from build123d import *

# Parameters (mm, degrees)
F0_W        = 28.575
F0_H        = 25.4
F1_DEPTH    = 3.175
F2_DEPTH    = 6.35
F3_T4_DEPTH = 58.0603739472
F6_DEPTH    = 25.4
F7_DEPTH    = 50.8


# Not quite as in the source:
# - a fillet or chamfer that OpenCascade refuses, or shapes differently, is made with other operations: its cross-section is extruded or revolved along the edge and cut away or added
# - a feature names something its author has since deleted; it is built from what else it names


with BuildPart() as f1:
    # F0 (on Top) → F1 (new body)
    with BuildSketch(Plane.XY):
        with Locations((14.2875, 0)):
            Rectangle(F0_W, F0_H)
        with BuildLine():
            Line((-9.525, -12.7), (0, -12.7))
            Line((0, -12.7), (0, 12.7))
            Line((0, 12.7), (-9.525, 12.7))
            Line((-9.525, 12.7), (-28.575, -4.1005208253))
            ThreePointArc((-28.575, -4.1005208253), (-25.0870430294, -7.374431916), (-21.0470880315, -9.9362869613))
            Line((-21.0470880315, -9.9362869613), (-10.525, -0.6566775598))
            Line((-10.525, -0.6566775598), (-11.1864378278, 0.0933224402))
            Line((-11.1864378278, 0.0933224402), (-21.3967655869, -8.9113402448))
            ThreePointArc((-21.3967655869, -8.9113402448), (-24.4613665471, -6.7728299311), (-27.1481868608, -4.1755232473))
            Line((-27.1481868608, -4.1755232473), (-9.525, 11.3666666667))
            Line((-9.525, 11.3666666667), (-9.525, -12.7))
        make_face()
    extrude(amount=F1_DEPTH)

    # F0 (on Top) → F2 (join)
    with BuildSketch(Plane.XY):
        with BuildLine():
            Line((-9.525, -12.7), (0, -12.7))
            Line((0, -12.7), (0, 12.7))
            Line((0, 12.7), (-9.525, 12.7))
            Line((-9.525, 12.7), (-28.575, -4.1005208253))
            ThreePointArc((-28.575, -4.1005208253), (-25.0870430294, -7.374431916), (-21.0470880315, -9.9362869613))
            Line((-21.0470880315, -9.9362869613), (-10.525, -0.6566775598))
            Line((-10.525, -0.6566775598), (-11.1864378278, 0.0933224402))
            Line((-11.1864378278, 0.0933224402), (-21.3967655869, -8.9113402448))
            ThreePointArc((-21.3967655869, -8.9113402448), (-24.4613665471, -6.7728299311), (-27.1481868608, -4.1755232473))
            Line((-27.1481868608, -4.1755232473), (-9.525, 11.3666666667))
            Line((-9.525, 11.3666666667), (-9.525, -12.7))
        make_face()
    extrude(amount=F2_DEPTH)

    # F3: chamfer of 6.35 on 1 edges, made by hand


with BuildPart() as f3_tool2:
    # F3_s3 → F3_t4 (new body)
    with BuildSketch(Plane.XZ.offset(29.0301869736)):
        Polygon((0, 0), (-6.35, 6.35), (0, 6.35), align=None)
    extrude(amount=-F3_T4_DEPTH)

    split(bisect_by=Plane.XY.offset(3.175), keep=Keep.TOP)


with BuildPart() as f1_1:
    add(f1.part)

    # F3_t1: cut F3_tool2
    add(f3_tool2.part, mode=Mode.SUBTRACT)

    # F5 (on face) → F6 (join)
    with BuildSketch(Plane(origin=(0, 12.7, 0), x_dir=(-1, 0, 0), z_dir=(0, 1, 0))):
        Polygon((3.175, 3.175), (-28.575, 3.175), (-28.575, 0), (9.525, 0), (9.525, 6.35), (6.35, 6.35), align=None)
        Polygon((-28.575, 0), (-28.575, 3.175), (-31.75, 3.175), align=None)
    extrude(amount=-F6_DEPTH)

    # F4 (on face) → F7 (cut)
    with BuildSketch(Plane(origin=(-9.525, 0, 0), x_dir=(0, -1, 0), z_dir=(-1, 0, 0))):
        Polygon((9.9561735988, 0), (12.7, 0), (12.7, 3.175), align=None)
    extrude(amount=-F7_DEPTH, mode=Mode.SUBTRACT)


solid = f1_1.part
Geometry: final body of the model. Coordinates: model frame, mm. A direction names the side the tool comes from. Give positions to 0.01 mm unless a question says otherwise; leave off trailing zeros. Write each loop counter-clockwise with the first axis right and the second up, starting at its lowest first coordinate (ties: lowest second). Pieces come first, ordered by that corner, then holes.
(1) Cut plane B-B, the plane z = 5.75. Return loops of the section in (x, y) (3 decimals), then the cut area to 3 significant figures.
(2) Ray query, line 1 (X direction, y = -4, z = 6) (3 decimals); line 2 (X direction, y = -1.25, z = 0.75) (3 decimals); line 3 (Z direction, x = 5.5, y = -8.5) (3 decimals). Return the intervals inside material, ascending.
(3) Cut plane C-C, the plane x = -4.5. Return loops of the section in (y, z) (3 decimals).
(4) Cut plane D-D, the plane y = 2. Return loops of the section in (x, z) (3 decimals).
(5) Cut plane A-A, the plane y = -7.5. Return loops of the section in (x, z) (3 decimals), then the cut area to 3 significant figures.
(6) Mould query, pull axis Y, two halves, no side actions, for faces 1 (the cylindrical face through (-25.14, -7.333, 3.131)), 2 (the flat face through (6, 2, 0)), 3 (the flat face through (-16.22, -4.346, 3.131)), 4 (the cylindrical face through (-24.421, -6.806, 3.131)). Classes: released by +Y, released by -Y, zero draft, split by the parting line, or undercut.
(7) Access query for faces 5 (the flat face through (-18.46, 3.487, 3.131)), 6 (the flat face through (14, 0, 3.175)), 7 (the flat face through (-9.525, 0, 3)). Directions: +Z, -Z, +X, -X, +Y, -Y. A direction counts if a zero-diameter tool reaches every point of the face in a straight line with its end or side. Return the directions, or none.
(8) First-contact query: P1, Ø10, axis at x = 20.5, y = 5.5, coming from the +Z side (3 decimals). Flat tip, straight axial feed; report the tip coordinate or a pass-through.
Values follow:
1. outline: (-28.575, -4.101) arc R25.4 ccw to (-21.047, -9.936) - (-10.525, -0.657) - (-11.186, 0.093) - (-21.397, -8.911) arc R23.498 cw to (-27.148, -4.176) - (-9.525, 11.367) - (-9.525, -12.7) - (-5.75, -12.7) - (-5.75, 12.7) - (-9.525, 12.7) - close
1. area: 142 mm2
2. line 1: x = -28.461 to -26.949, -15.828 to -14.316, -9.525 to -6
2. line 2: x = -25.343 to -23.831, -12.71 to -11.198, -9.525 to 29.325
2. line 3: z = 0 to 3.175
3. outline: (-12.7, 3.175) - (-9.956, 0) - (12.7, 0) - (12.7, 4.5) - (-12.7, 4.5) - close
4. outline: (-21.658, 0) - (-20.146, 0) - (-20.146, 6.35) - (-21.658, 6.35) - close; (-9.525, 0) - (28.575, 0) - (31.75, 3.175) - (-3.175, 3.175) - (-6.35, 6.35) - (-9.525, 6.35) - close
5. outline: (-24.924, 0) - (-23.532, 0) - (-23.532, 6.35) - (-24.924, 6.35) - close; (-19.796, 0) - (-18.285, 0) - (-18.285, 6.35) - (-19.796, 6.35) - close; (-9.525, 0) - (28.575, 0) - (31.75, 3.175) - (-3.175, 3.175) - (-6.35, 6.35) - (-9.525, 6.35) - close
5. area: 160 mm2
6. face 1: released by -Y
6. face 2: zero draft
6. face 3: undercut
6. face 4: undercut
7. face 5: +Z, -Z
7. face 6: +Z, +X, +Y, -Y
7. face 7: +Z, -Z, -Y
8. P1: stops at z = 3.175
